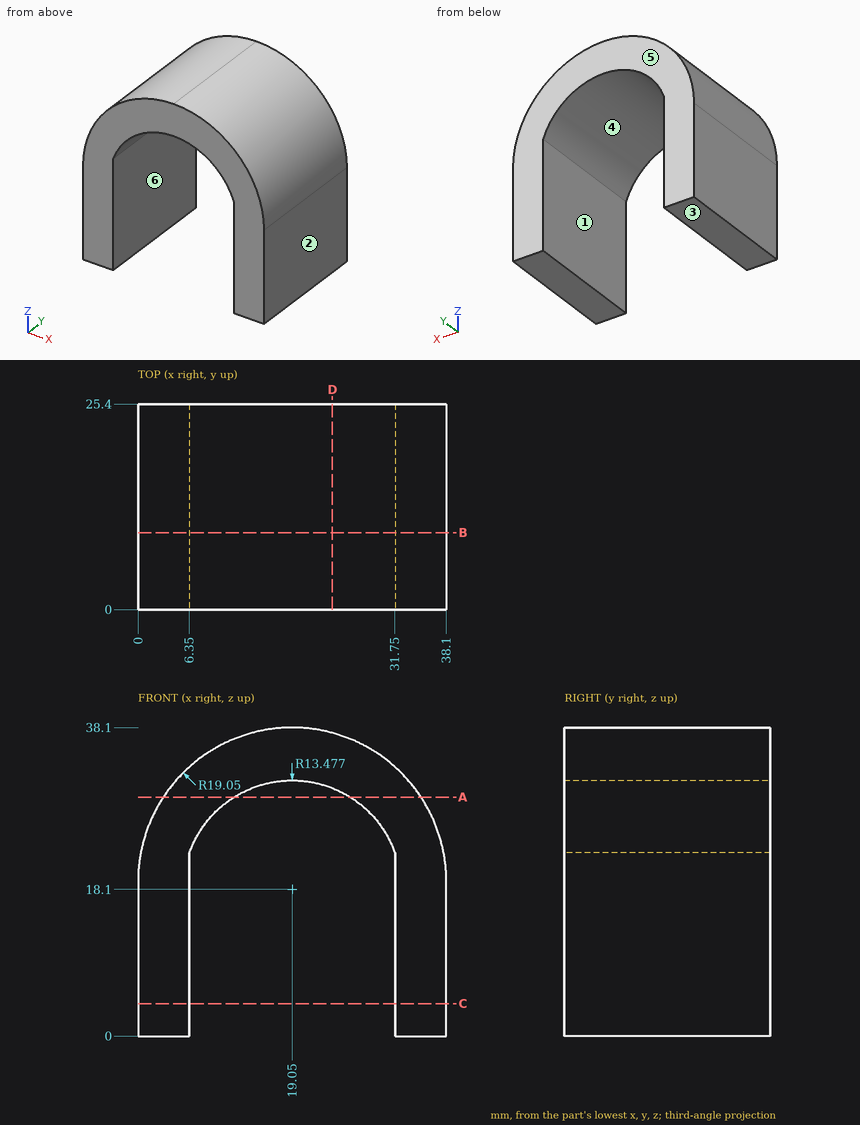
Source: three-view drawing plus pictorial views. Frame: mm from the lowest corner of the part. A direction names the side the tool comes from. Round coordinates to 2 decimals unless told otherwise and drop trailing zeros. Order: outer loops, then holes, each group sorted by start corner. A loop starts at its lowest first (then second) coordinate and runs counter-clockwise, first axis right, second up. Notation, with made-up numbers: (60.25, -23) -> (72.25, -23) arc R17 cw to (72.25, -1) -> close; hole circle Ø5 at (51.25, 51.5). An arc over 180 degrees is marked (long way). Use one line per item in the form item = value. Start each with the question number.
1. Pin query (flat end, axial travel): pin 1 Ø6 at (y, z) = (22.5, 25.5) entering from +X (1 decimal); pin 2 Ø6 at (x, y) = (4, 15.5) entering from +Z (1 decimal); pin 3 Ø3 at (x, z) = (7, 19.5) entering from +Y; pin 4 Ø4 at (x, y) = (27.5, 5) entering from -Z. Return the tip coordinate at first contact, or that it passes through.
2. Cut plane D-D (x = 24). Return the cut outline in (y, z) (1 decimal).
3. Reachability of the marked faces 5 and 6 from +Z, -Z, +X, -X, +Y, -Y: full face, straight path, thin tool, end or side. Return the list, or none.
4. Line query: probe 1 along X at (y, z) = (17.5, 8); probe 2 along X at (y, z) = (19.25, 25.5) (1 decimal); probe 3 along X at (y, z) = (15.5, 33) (1 decimal). Output: solid intervals per line, ascending.
5. Draft query along X for the marked faces 1, 2, 3 and 4. Return one class per face: pulls with the +X half, pulls with the -X half, needs draft (parallel to the pull), parting line crosses it, or undercut.
6. Cut plane A-A (z = 29.5). Return the cut outline in (x, y), then the cut area to 3 significant figures.
7. Cut plane B-B (y = 9.5). Return the cut outline in (x, z).
8. Cut plane C-C (z = 4). Return the cut outline in (x, y).
Solution:
q1.pin_1 = 37.8
q1.pin_2 = 33.8
q1.pin_3 = 25.4
q1.pin_4 = 26.61
q2.outline = (0, 30.6) -> (25.4, 30.6) -> (25.4, 37.4) -> (0, 37.4) -> close
q3.face_5 = +Z, -Z, +X, -X, +Y
q3.face_6 = -Z, +Y, -Y
q4.probe_1 = 0 to 6.35, 31.75 to 38.1
q4.probe_2 = 1.1 to 7.8, 30.3 to 37
q4.probe_3 = 6.1 to 32
q5.face_1 = undercut
q5.face_2 = pulls with the +X half
q5.face_3 = needs draft
q5.face_4 = undercut
q6.outline = (3.12, 0) -> (11.86, 0) -> (11.86, 25.4) -> (3.12, 25.4) -> close; (26.24, 0) -> (34.98, 0) -> (34.98, 25.4) -> (26.24, 25.4) -> close
q6.area = 444 mm^2
q7.outline = (0, 0) -> (6.35, 0) -> (6.35, 22.61) arc R13.48 cw to (31.75, 22.61) -> (31.75, 0) -> (38.1, 0) -> (38.1, 19.05) arc R19.05 ccw to (19.05, 38.1) arc R19.05 ccw to (0, 19.05) -> close
q8.outline = (0, 0) -> (6.35, 0) -> (6.35, 25.4) -> (0, 25.4) -> close; (31.75, 0) -> (38.1, 0) -> (38.1, 25.4) -> (31.75, 25.4) -> close
